Job drawing, mm, ordinate dimensions from the low corner. One solid piece. Give positions to 0.01 mm unless a question says otherwise; leave off trailing zeros. Order: outer loops, then holes, each group sorted by start corner. A loop starts at its lowest first (then second) coordinate and runs counter-clockwise, first axis right, second up. Notation, with made-up numbers: (40.25, -4) -> (53.25, -4) arc R11 cw to (53.25, 6) -> close; hole circle Ø6 at (-5.5, 11). An arc over 180 degrees is marked (long way). Write item = value, one per line. Start each with the question number.
(1) Probe line 1 along Y through (x, z) = (34, 0.75); line 2 along X through (y, z) = (91.4, 1); line 3 along X through (y, z) = (78.9, 0.95). List the from-to ranges inside material, lowest first. Write a range as from..to.
(2) Saw through at A-A, the plane y = 35.4. List the corners of the cut face in (x, z), then the cut area to 3 significant figures.
(3) Saw through at B-B, the plane z = 1.7. State how many separate pieces and enclosed holes the cut face has, then the cut area to 3 significant figures.
(4) Flat gauge pin, fed straight in: pin 1 (1 mm diameter, centred on x = 12.5, z = 1, fed in from -Y). Where does the tip first touch, or does it go through?
(5) Saw through at C-C, the plane y = 71.4. List the corners of the cut face in (x, z).
(6) Saw through at D-D, the plane x = 23. List the corners of the cut face in (y, z), then the cut area to 3 significant figures.
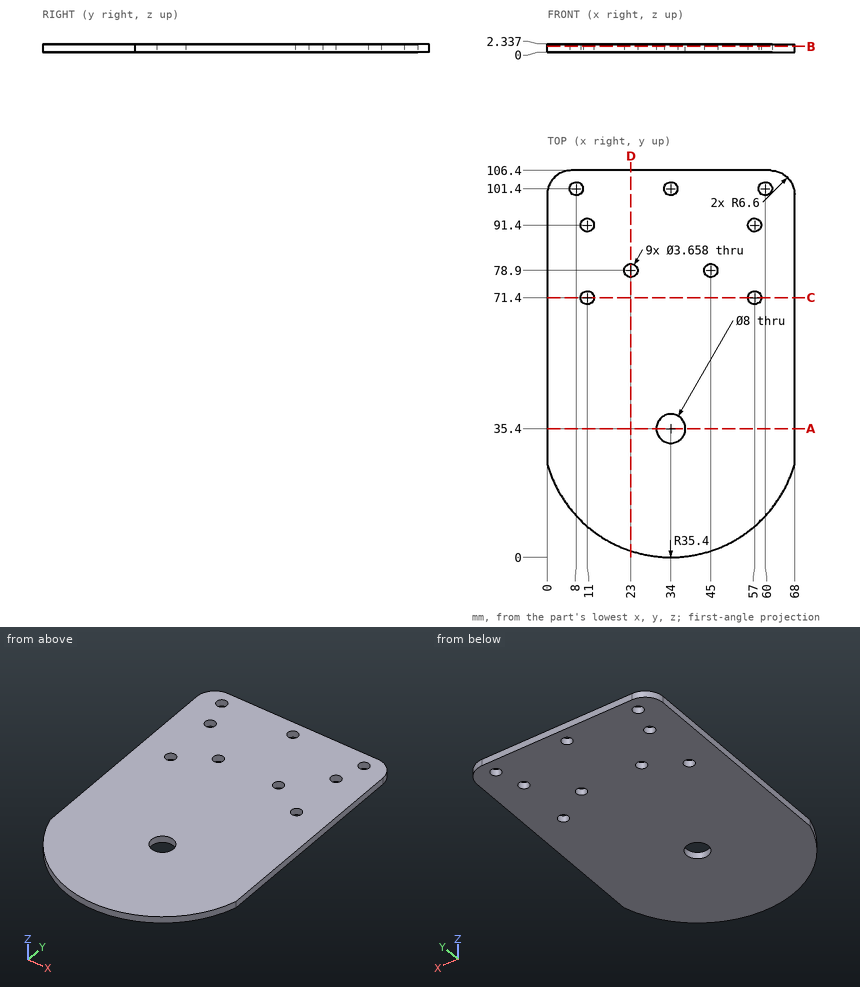
Results list:
q1.line_1 = 0..31.4, 39.4..99.57, 103.23..106.4
q1.line_2 = 0..9.17, 12.83..55.17, 58.83..68
q1.line_3 = 0..21.17, 24.83..43.17, 46.83..68
q2.outline = (0, 0) -> (30, 0) -> (30, 2.34) -> (0, 2.34) -> close; (38, 0) -> (68, 0) -> (68, 2.34) -> (38, 2.34) -> close
q2.area = 140 mm^2
q3.separate_pieces = 1
q3.enclosed_holes = 10
q3.area = 6,610 mm^2
q4.pin_1 = 6.9
q5.outline = (0, 0) -> (9.17, 0) -> (9.17, 2.34) -> (0, 2.34) -> close; (12.83, 0) -> (55.17, 0) -> (55.17, 2.34) -> (12.83, 2.34) -> close; (58.83, 0) -> (68, 0) -> (68, 2.34) -> (58.83, 2.34) -> close
q6.outline = (1.75, 0) -> (77.07, 0) -> (77.07, 2.34) -> (1.75, 2.34) -> close; (80.73, 0) -> (106.4, 0) -> (106.4, 2.34) -> (80.73, 2.34) -> close
q6.area = 236 mm^2
